Verification items for the finished model (mm, model axes). Face numbers are marked on the shaded views. A direction names the side the tool comes from. Coordinates: 2 decimals unless noted, no trailing zeros. Loops run counter-clockwise (first coordinate to the right, second up) from the corner with the lowest first, then second, coordinate; pieces in that order, holes last. Notation, with made-up numbers: M 33.5,47.25 L 38.5,47.25 A21 cw 38.5,73.25 Z; hole C 60,7 d3. An arc over 180 degrees is marked long. Write item = value, one per line. Start each with the question number.
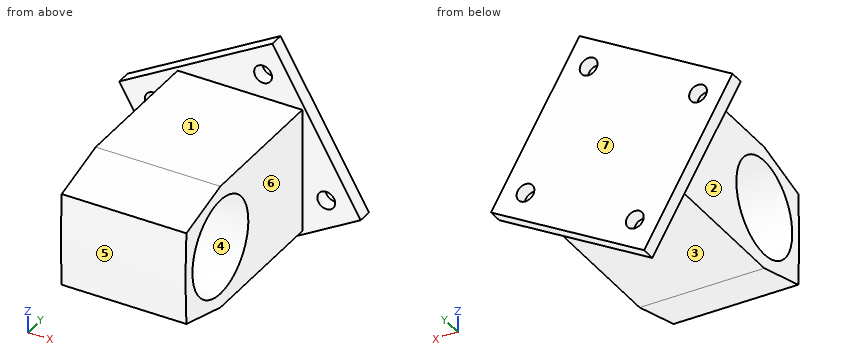
```python
from build123d import *

# Parameters (mm, degrees)
SKETCH1_W           = 44.45
SKETCH1_H           = 44.45
BOSS_EXTRUDE1_DEPTH = 50.292
BOSS_EXTRUDE2_DEPTH = 44.45
SKETCH3_R           = 17.145
CUT_EXTRUDE1_DEPTH  = 127
BOSS_EXTRUDE3_DEPTH = 5.08
SKETCH5_R           = 3.175
CUT_EXTRUDE2_DEPTH  = 77.68803402


with BuildPart() as part:
    # Sketch1 → Boss-Extrude1 (new body)
    with BuildSketch(Plane(origin=(0, 0, 0), x_dir=(1, 0, 0), z_dir=(0, 1, 0))):
        Rectangle(SKETCH1_W, SKETCH1_H)
    extrude(amount=BOSS_EXTRUDE1_DEPTH)

    # Sketch2 → Boss-Extrude2 (add)
    with BuildSketch(Plane(origin=(22.225, 0, 0), x_dir=(0, 0, -1), z_dir=(1, 0, 0))):
        with BuildLine():
            Line((-22.225, 0), (-16.637096816, -20.85433859))
            ThreePointArc((-16.637096816, -20.85433859), (0, -21.31603402), (16.637096816, -20.85433859))
            Line((16.637096816, -20.85433859), (22.225, 0))
            Line((22.225, 0), (-22.225, 0))
        make_face()
    extrude(amount=-BOSS_EXTRUDE2_DEPTH)

    # Sketch3 → Cut-Extrude1 (cut)
    with BuildSketch(Plane(origin=(22.225, 0, 0), x_dir=(0, 0, -1), z_dir=(1, 0, 0))):
        Circle(SKETCH3_R)
    extrude(amount=-CUT_EXTRUDE1_DEPTH, mode=Mode.SUBTRACT)

    # Sketch4 → Boss-Extrude3 (add)
    with BuildSketch(Plane(origin=(0, 50.292, 0), x_dir=(1, 0, 0), z_dir=(0, 1, 0))):
        Polygon((43.024336118, 11.528336118), (11.528336118, -43.024336118), (-43.024336118, -11.528336118), (-11.528336118, 43.024336118), align=None)
    extrude(amount=BOSS_EXTRUDE3_DEPTH)

    # Sketch5 → Cut-Extrude2 (cut, through all)
    with BuildSketch(Plane(origin=(0, 55.372, 0), x_dir=(1, 0, 0), z_dir=(0, 1, 0))):
        with Locations((30.757078124, 8.241334245)):
            Circle(SKETCH5_R)
        with Locations((8.241334245, -30.757078124)):
            Circle(SKETCH5_R)
        with Locations((-8.241334245, 30.757078124)):
            Circle(SKETCH5_R)
        with Locations((-30.757078124, -8.241334245)):
            Circle(SKETCH5_R)
    extrude(amount=-CUT_EXTRUDE2_DEPTH, mode=Mode.SUBTRACT)


solid = part.part
```
Q1. Sectioned sample at B-B on y = 3. Record the cut outline in (x, z) (1 decimal).
Q2. Sectioned sample at D-D on x = 20. Record the cut outline in (y, z) (3 decimals).
Q3. Sectioned sample at A-A on z = -14. Record the cut outline in (x, y) (3 decimals).
Q4. Scan lines: L1, parallel to Y at x = -25, z = -4; L2, parallel to Y at x = -3, z = 0 (3 decimals); L3, parallel to Y at x = -11.5, z = 14.5. Record each from-to range of solid material in increasing order. Write a range as [from, to].
Q5. Sectioned sample at C-C on x = 30. Record the cut outline in (y, z).
Q6. Set-up check for the marked faces 1, 2 and 3: record each of +Z, -Z, +X, -X, +Y, -Y from which the full face is reachable in a straight line by a thin tool's end or side.
Q7. Gauge pin test, flat ends, axial feed: pin 1 (10 mm diameter, centred on y = 28.5, z = -25.5, fed in from -X) (3 decimals); pin 2 (7.5 mm diameter, centred on x = -30.76, z = 8.24, fed in from -Y); pin 3 (10 mm diameter, centred on y = 43, z = 19.5, fed in from +X) (3 decimals). Record the tip position at first contact, or that the pin passes through.
Q8. Mould release check, pull along Y, two halves, no side actions. Record for the marked faces 4, 5, 6 and 7: +Y half, -Y half, draft (parallel to the pull), parting line (faces both ways), or undercut.
Solutions:
q1.outline = M -22.2,-22.2 L 22.2,-22.2 L 22.2,-16.9 L -22.2,-16.9 Z; M -22.2,16.9 L 22.2,16.9 L 22.2,22.2 L -22.2,22.2 Z
q2.outline = M -20.854,-16.637 L 0,-22.225 L 50.292,-22.225 L 50.292,-24.821 L 55.372,-24.821 L 55.372,28.351 L 50.292,28.351 L 50.292,22.225 L 0,22.225 L -20.854,16.637 A299.988 ccw Z; hole C 0,0 d34.29
q3.outline = M -28.286,50.292 L -22.225,50.292 L -22.225,9.897 L 22.225,9.897 L 22.225,50.292 L 38.743,50.292 L 38.743,55.372 L -28.286,55.372 Z; M -22.225,-20.989 L 22.225,-20.989 L 22.225,-9.897 L -22.225,-9.897 Z
q4.L1 = [50.29, 55.37]
q4.L2 = [-21.316, -17.145], [17.145, 55.372]
q4.L3 = [-20.97, -9.15], [9.15, 55.37]
q5.outline = M 50.29,-19.05 L 55.37,-19.05 L 55.37,-11.32 L 50.29,-11.32 Z; M 50.29,-5.16 L 55.37,-5.16 L 55.37,11.03 L 50.29,11.03 Z
q6.face_1 = +Z, +X, -X, -Y
q6.face_2 = +Z, -Z, -X, -Y
q6.face_3 = -Z, +X, -X, -Y
q7.pin_1 = -22.225
q7.pin_2 = 50.29
q7.pin_3 = 22.225
q8.face_4 = undercut
q8.face_5 = -Y half
q8.face_6 = draft
q8.face_7 = +Y half
